The drawing under review shows one solid part. Ordinate dimensions are in mm from its lowest x, y, z. Coordinates: 2 decimals unless noted, no trailing zeros. Write each loop counter-clockwise with the first axis right and the second up, starting at its lowest first coordinate (ties: lowest second). Pieces come first, ordered by that corner, then holes.
Q1. Add section B-B, the plane y = 1.25. Give the boundary of the cut face in (x, z).
Q2. Add section D-D, the plane y = 4.5. Give the boundary of the cut face in (x, z).
Q3. Add section C-C, the plane z = 18.25. Give the number of separate pieces and of enclosed holes in the cut face, plus the area to 3 significant figures.
Q4. Add section A-A, the plane x = 19.05. Give the boundary of the cut face in (y, z), plus the area to 3 significant figures.
Q5. To check wall thickness, follow probe 1 along X at (y, z) = (4.75, 12.5) (1 decimal); probe 2 along X at (y, z) = (1.5, 20.5) (1 decimal); probe 3 along Z at (x, y) = (55.5, 4.25). State the ranges of each line that lie inside material, in increasing order.
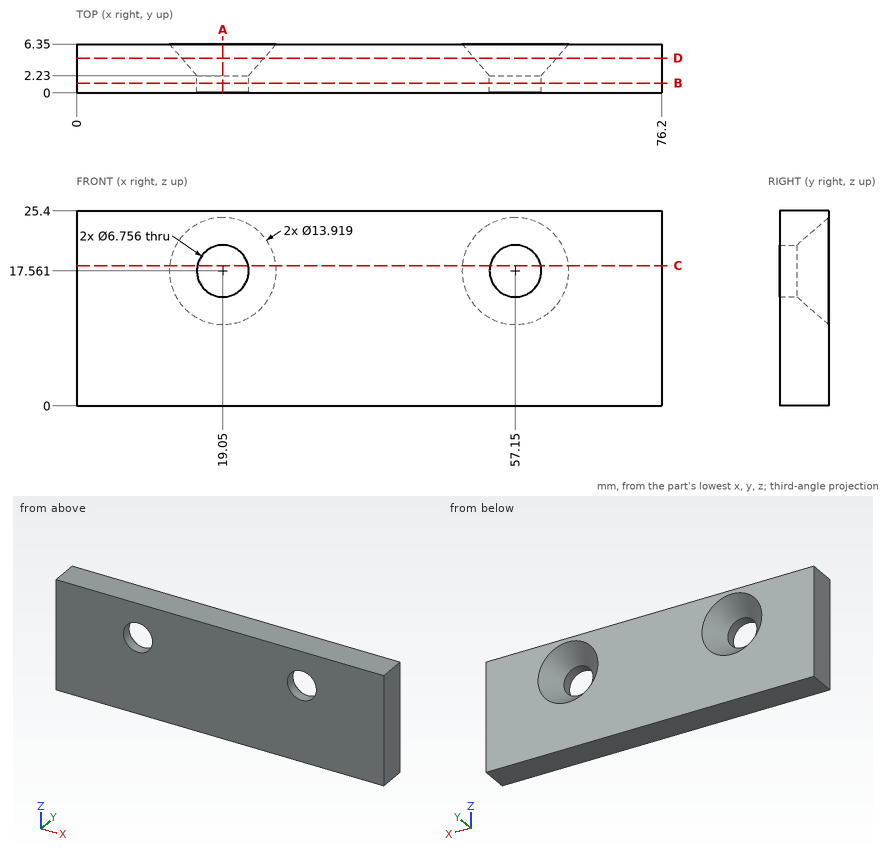
Here are the results:
1. outline: (0, 0) - (76.2, 0) - (76.2, 25.4) - (0, 25.4) - close; hole circle Ø6.76 at (19.05, 17.56); hole circle Ø6.76 at (57.15, 17.56)
2. outline: (0, 0) - (76.2, 0) - (76.2, 25.4) - (0, 25.4) - close; hole circle Ø10.7 at (19.05, 17.56); hole circle Ø10.7 at (57.15, 17.56)
3. separate pieces: 3
3. enclosed holes: 0
3. area: 370 mm2
4. outline: (0, 0) - (6.35, 0) - (6.35, 10.6) - (2.23, 14.18) - (0, 14.18) - close; (0, 20.94) - (2.23, 20.94) - (6.35, 24.52) - (6.35, 25.4) - (0, 25.4) - close
4. area: 104 mm2
5. probe 1: x = 0 to 16.7, 21.4 to 54.8, 59.5 to 76.2
5. probe 2: x = 0 to 17.4, 20.7 to 55.5, 58.8 to 76.2
5. probe 3: z = 0 to 12.7, 22.42 to 25.4
